```python
from build123d import *

# Parameters (mm, degrees)
CYLINDER178_R     = 2
CYLINDER178_DEPTH = 20
CYLINDER177_R     = 2
CYLINDER177_DEPTH = 20
CYLINDER175_R     = 2
CYLINDER175_DEPTH = 20
CYLINDER176_R     = 2
CYLINDER176_DEPTH = 20
BOX069_W          = 38.8
BOX069_H          = 40.1
BOX069_DEPTH      = 20.1
BOX084_W          = 2.7
BOX084_H          = 54
BOX084_DEPTH      = 20.1


with BuildPart() as cylinder178:
    # Cylinder178 → Cylinder178 (new body)
    with BuildSketch(Plane(origin=(-97.2, -71.8, 5), x_dir=(0, 0, -1), z_dir=(1, 0, 0))):
        Circle(CYLINDER178_R)
    extrude(amount=CYLINDER178_DEPTH)


with BuildPart() as cylinder177:
    # Cylinder177 → Cylinder177 (new body)
    with BuildSketch(Plane(origin=(-97.2, -71.8, 15), x_dir=(0, 0, -1), z_dir=(1, 0, 0))):
        Circle(CYLINDER177_R)
    extrude(amount=CYLINDER177_DEPTH)


with BuildPart() as cylinder175:
    # Cylinder175 → Cylinder175 (new body)
    with BuildSketch(Plane(origin=(-97.2, -22.1, 5), x_dir=(0, 0, -1), z_dir=(1, 0, 0))):
        Circle(CYLINDER175_R)
    extrude(amount=CYLINDER175_DEPTH)


with BuildPart() as cylinder176:
    # Cylinder176 → Cylinder176 (new body)
    with BuildSketch(Plane(origin=(-97.2, -22.1, 15), x_dir=(0, 0, -1), z_dir=(1, 0, 0))):
        Circle(CYLINDER176_R)
    extrude(amount=CYLINDER176_DEPTH)


with BuildPart() as box069:
    # Box069 → Box069 (new body)
    with BuildSketch(Plane(origin=(82, -93, 0), x_dir=(1, 0, 0), z_dir=(0, 0, 1))):
        with Locations((19.4, 20.05)):
            Rectangle(BOX069_W, BOX069_H)
    extrude(amount=BOX069_DEPTH)


with BuildPart() as cut131:
    # Box084 → Box084 (new body)
    with BuildSketch(Plane(origin=(90.8, -99.95, 0), x_dir=(1, 0, 0), z_dir=(0, 0, 1))):
        with Locations((1.35, 27)):
            Rectangle(BOX084_W, BOX084_H)
    extrude(amount=BOX084_DEPTH)

    # Fusion084: union Box069
    add(box069.part)


with BuildPart() as cut131_1:
    # Fusion084 placement: moved
    add(cut131.part.moved(Location((-188, 26, 0))))

    # Cut128: cut Cylinder176
    add(cylinder176.part, mode=Mode.SUBTRACT)

    # Cut129: cut Cylinder175
    add(cylinder175.part, mode=Mode.SUBTRACT)

    # Cut130: cut Cylinder177
    add(cylinder177.part, mode=Mode.SUBTRACT)

    # Cut131: cut Cylinder178
    add(cylinder178.part, mode=Mode.SUBTRACT)


with BuildPart() as cut131_2:
    # Cut131 placement: moved
    add(cut131_1.part.moved(Location((4, 10, 0))))


solid = cut131_2.part
```
Here's how the part is built. I have some questions about the finished solid (model axes, mm). A direction names the side the tool comes from. Coordinates: 2 decimals unless noted, no trailing zeros. Write each loop counter-clockwise with the first axis right and the second up, starting at its lowest first coordinate (ties: lowest second). Pieces come first, ordered by that corner, then holes. Notation, with made-up numbers: M -23.75,-39.5 L -5.75,-39.5 A18 ccw -5.75,-16.5 Z; hole C 79,-29.75 d10. An arc over 180 degrees is marked long. Answer as CSV lines item,"result". Start each with the question number.
Q1. For faces 1 (the flat face through (-93.2, -61, 10)), 2 (the flat face through (-98, -16.9, 10)), 3 (the flat face through (-90.5, -61, 10)), 4 (the flat face through (-77, -16.9, 10)), which set-ups out of +Z, -Z, +X, -X, +Y, -Y let a thin tool reach every point of the face, with its end or its side?
Q2. Suppose I cut it at C-C, the plane z = 15. List the corners of the cut face in (x, y) for me.
Q3. Suppose I cut it at A-A, the plane y = -12.1. List the corners of the cut face in (x, z) for me, then the cut area to 3 significant figures.
Q4. I need wall thicknesses on probe 1 along Z at (x, y) = (-91, -12); probe 2 along Y at (x, z) = (-91.65, 5); probe 3 along Z at (x, y) = (-91, -61). Which ranges of each line are inside material? Lowest first, please. Write a range as [from, to].
Q5. Will these pins go through, and if not, where does the flat tip stop? pin 1 Ø2.5 at (x, z) = (-99, 9.5) entering from -Y; pin 2 Ø8 at (x, y) = (-93, -57) entering from -Z; pin 3 Ø6 at (x, z) = (-67.5, 7.5) entering from +Y; pin 4 Ø4.5 at (y, z) = (-12.1, 15) entering from +X.
Q6. Suppose I cut it at B-B, the plane x = -92. List the corners of the cut face in (y, z) for me.
Q7. Suppose I cut it at D-D, the plane z = 9.25. List the corners of the cut face in (x, y) for me.
Q8. If we mould it in two halves opening along Z, with no side actions, what happens to faces 5 (the flat face through (-90.5, -13, 10)), 6 (the cylindrical face through (-91.869, -60.448, 6.474)), 7 (the flat face through (-83, -37, 0))? For each: pulls with the +Z half, pulls with the -Z half, needs draft (parallel to the pull), parting line crosses it, or undercut.
Entries:
1,face 1,"+Z, -Z, -X, -Y"
1,face 2,"+Z, -Z, -X, +Y"
1,face 3,"+Z, -Z, +X, -Y"
1,face 4,"+Z, -Z, +X, +Y"
2,outline,"M -102,-57 L -93.2,-57 L -93.2,-59.8 L -90.5,-59.8 L -90.5,-57 L -63.2,-57 L -63.2,-16.9 L -90.5,-16.9 L -90.5,-14.1 L -93.2,-14.1 L -93.2,-16.9 L -102,-16.9 Z; M -93.2,-63.95 L -90.5,-63.95 L -90.5,-63.8 L -93.2,-63.8 Z; M -93.2,-10.1 L -90.5,-10.1 L -90.5,-9.95 L -93.2,-9.95 Z"
3,outline,"M -93.2,0 L -90.5,0 L -90.5,3 L -93.2,3 Z; M -93.2,7 L -90.5,7 L -90.5,13 L -93.2,13 Z; M -93.2,17 L -90.5,17 L -90.5,20.1 L -93.2,20.1 Z"
3,area,"32.7 mm²"
4,probe 1,"z = [0, 3], [7, 13], [17, 20.1]"
4,probe 2,"y = [-63.95, -63.8], [-59.8, -14.1], [-10.1, -9.95]"
4,probe 3,"z = [0, 3.17], [6.83, 13.17], [16.83, 20.1]"
5,pin 1,"stops at y = -57"
5,pin 2,"stops at z = 0"
5,pin 3,"stops at y = -16.9"
5,pin 4,"stops at x = -90.5"
6,outline,"M -63.95,0 L -9.95,0 L -9.95,20.1 L -63.95,20.1 Z; hole C -61.8,5 d4; hole C -61.8,15 d4; hole C -12.1,5 d4; hole C -12.1,15 d4"
7,outline,"M -102,-57 L -93.2,-57 L -93.2,-63.95 L -90.5,-63.95 L -90.5,-57 L -63.2,-57 L -63.2,-16.9 L -90.5,-16.9 L -90.5,-9.95 L -93.2,-9.95 L -93.2,-16.9 L -102,-16.9 Z"
8,face 5,"needs draft"
8,face 6,"undercut"
8,face 7,"pulls with the -Z half"
